Check sheet for the drawn part. Datum: minimum x, y, z corner. Units: mm. A direction names the side the tool comes from. Coordinates: 2 decimals unless noted, no trailing zeros. Write each loop counter-clockwise with the first axis right and the second up, starting at its lowest first coordinate (ties: lowest second). Pieces come first, ordered by that corner, then holes. Notation, with made-up numbers: (-12, -3) -> (-3, -3) arc R4 ccw to (-3, 2) -> close; hole circle Ø8 at (-30, -11.5). An arc over 180 degrees is marked (long way). One line per question, with ' | ' between items.
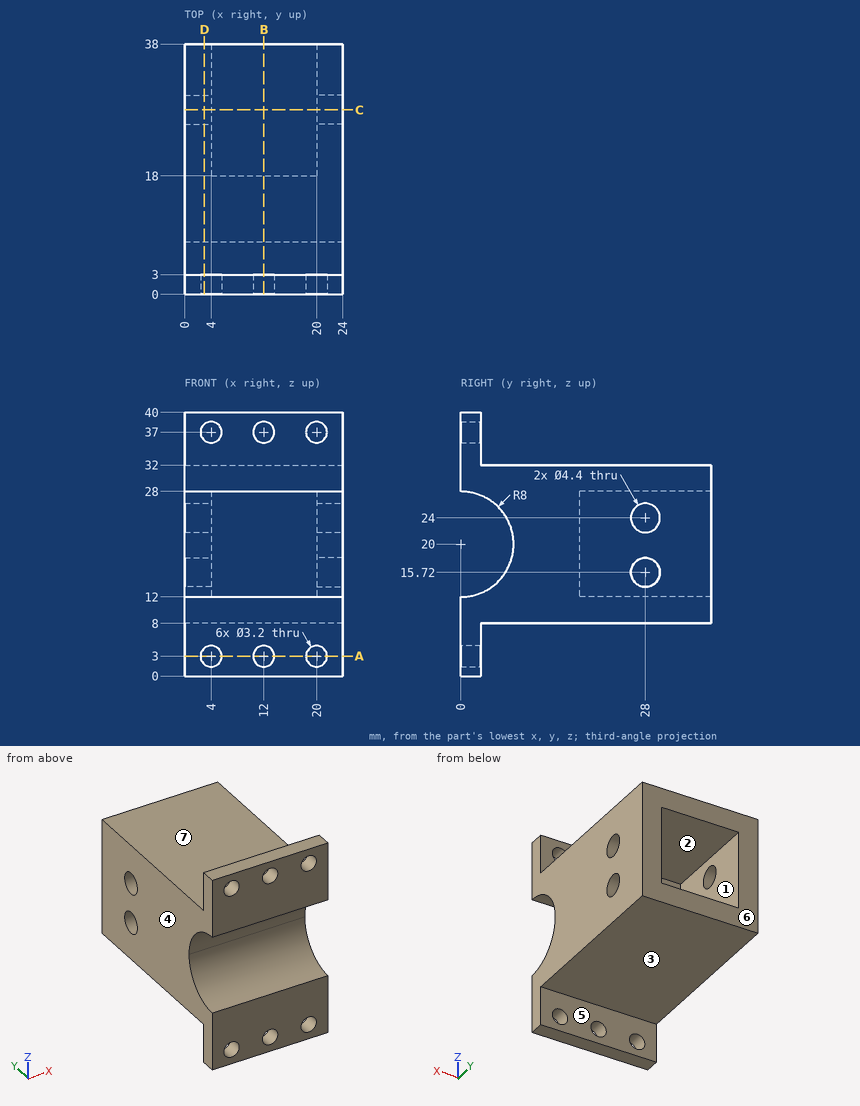
1. Cross-section at C-C on y = 28. Record the boundary of the cut face in (x, z), and give its area (3 significant figures).
Worked answers:
outline: (0, 8) -> (24, 8) -> (24, 13.52) -> (20, 13.52) -> (20, 12) -> (4, 12) -> (4, 13.52) -> (0, 13.52) -> close; (0, 17.92) -> (4, 17.92) -> (4, 21.8) -> (0, 21.8) -> close; (0, 26.2) -> (4, 26.2) -> (4, 28) -> (20, 28) -> (20, 26.2) -> (24, 26.2) -> (24, 32) -> (0, 32) -> close; (20, 17.92) -> (24, 17.92) -> (24, 21.8) -> (20, 21.8) -> close | area: 250 mm²
2. Go/stop test with flat-tipped pins: P1, Ø8, axis at x = 15, y = 32.5, coming from the +Z side; P2, Ø13, axis at x = 11.5, y = 29, coming from the -Z side; P3, Ø5, axis at x = 20, z = 3, coming from the +Y side. Record where each tip stops, or that it passes through.
Worked answers:
P1: z = 32 | P2: z = 8 | P3: y = 3
3. Cross-section at A-A on z = 3. Record the boundary of the cut face in (x, y).
Worked answers:
outline: (0, 0) -> (2.4, 0) -> (2.4, 3) -> (0, 3) -> close; (5.6, 0) -> (10.4, 0) -> (10.4, 3) -> (5.6, 3) -> close; (13.6, 0) -> (18.4, 0) -> (18.4, 3) -> (13.6, 3) -> close; (21.6, 0) -> (24, 0) -> (24, 3) -> (21.6, 3) -> close
4. Material ranges on line 1 (X direction, y = 2.2, z = 3); line 2 (X direction, y = 19, z = 14); line 3 (Z direction, x = 7.5, y = 31.5), recorded low to high. Write a range as from..to.
Worked answers:
line 1: 0..2.4, 5.6..10.4, 13.6..18.4, 21.6..24 | line 2: 0..4, 20..24 | line 3: 8..12, 28..32
5. Cross-section at D-D on x = 3. Record the boundary of the cut face in (y, z).
Worked answers:
outline: (0, 0) -> (3, 0) -> (3, 1.75) -> (0, 1.75) -> close; (0, 4.25) -> (3, 4.25) -> (3, 8) -> (38, 8) -> (38, 32) -> (3, 32) -> (3, 35.75) -> (0, 35.75) -> (0, 28) arc R8 cw to (0, 12) -> close; (0, 38.25) -> (3, 38.25) -> (3, 40) -> (0, 40) -> close; hole circle Ø4.4 at (28, 15.72); hole circle Ø4.4 at (28, 24)
6. Mould release check, pull along X, two halves, no side actions. Record for the marked faces 1, 2, 3 and 4: released by +X, released by -X, zero draft, split by the parting line, or undercut.
Worked answers:
face 1: undercut | face 2: undercut | face 3: zero draft | face 4: released by -X
7. Cross-section at B-B on x = 12. Record the boundary of the cut face in (y, z), and give its area (3 significant figures).
Worked answers:
outline: (0, 0) -> (3, 0) -> (3, 1.4) -> (0, 1.4) -> close; (0, 4.6) -> (3, 4.6) -> (3, 8) -> (38, 8) -> (38, 12) -> (18, 12) -> (18, 28) -> (38, 28) -> (38, 32) -> (3, 32) -> (3, 35.4) -> (0, 35.4) -> (0, 28) arc R8 cw to (0, 12) -> close; (0, 38.6) -> (3, 38.6) -> (3, 40) -> (0, 40) -> close | area: 520 mm²
8. Tool access check on the marked faces 5, 6 and 7. Record the directions out of +Z, -Z, +X, -X, +Y, -Y that give a thin tool (end or side, any length) a straight path to the whole face; none if there is none.
Worked answers:
face 5: -Z, +X, -X, +Y | face 6: +Z, -Z, +X, -X, +Y | face 7: +Z, +X, -X, +Y
